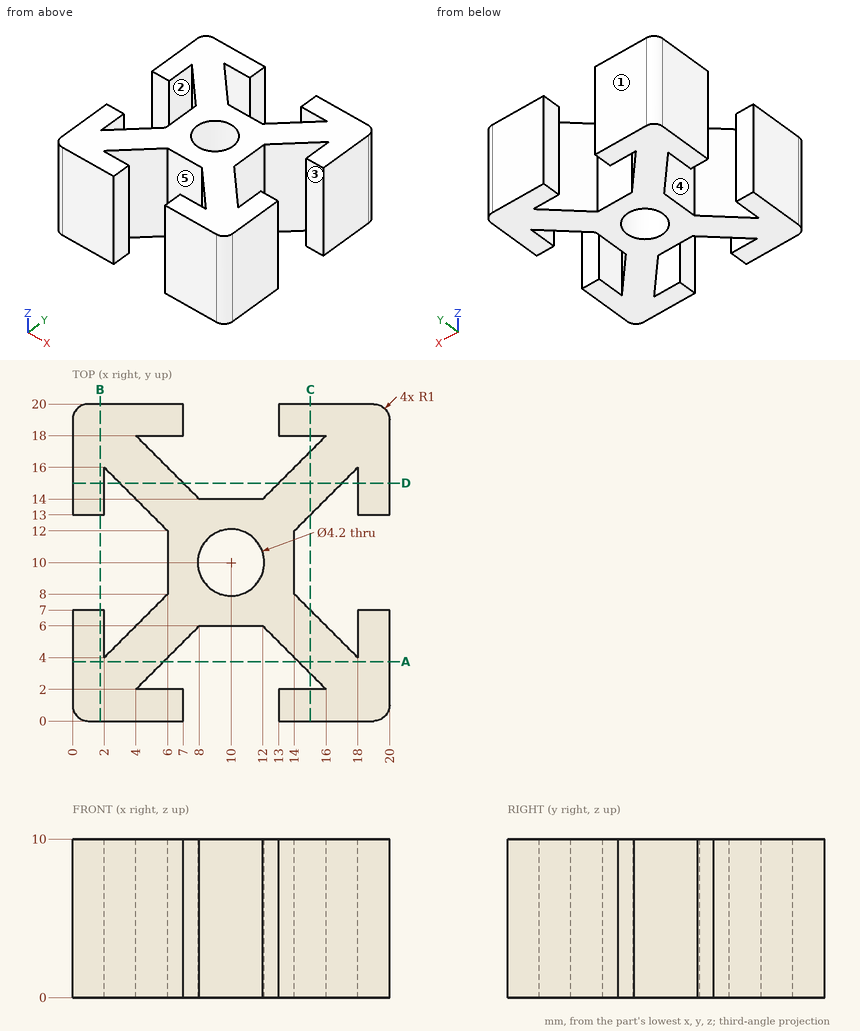
The figure shows three views and two pictorial views of one solid part (mm, origin at its lowest corner). Answer the questions. A direction names the side the tool comes from. Give positions to 0.01 mm unless a question says otherwise; leave off trailing zeros. Write each loop counter-clockwise with the first axis right and the second up, starting at its lowest first coordinate (ties: lowest second). Pieces come first, ordered by that corner, then holes. Notation, with made-up numbers: (12.25, -16.75) - (50.25, -16.75) arc R25 cw to (50.25, 19.25) - close; hole circle Ø7 at (44.25, 44.5). An arc over 180 degrees is marked (long way). Return JSON: item names as keys, results as strings.
Q1. A cutting plane is placed at A-A, the plane y = 3.75. Determine the outline of the cut face in (x, z).
Reply:
{"outline": "(0, 0) - (5.75, 0) - (5.75, 10) - (0, 10) - close; (14.25, 0) - (20, 0) - (20, 10) - (14.25, 10) - close"}
Q2. A cutting plane is placed at B-B, the plane x = 1.75. Determine the outline of the cut face in (y, z).
Reply:
{"outline": "(0, 0) - (7, 0) - (7, 10) - (0, 10) - close; (13, 0) - (20, 0) - (20, 10) - (13, 10) - close"}
Q3. A cutting plane is placed at C-C, the plane x = 15. Determine the outline of the cut face in (y, z).
Reply:
{"outline": "(0, 0) - (2, 0) - (2, 10) - (0, 10) - close; (3, 0) - (7, 0) - (7, 10) - (3, 10) - close; (13, 0) - (17, 0) - (17, 10) - (13, 10) - close; (18, 0) - (20, 0) - (20, 10) - (18, 10) - close"}
Q4. Consider line 1 along X through (y, z) = (5.25, 9.75); line 2 along Y through (x, z) = (15.25, 4.5). Determine where each line is inside the solid, lowest interval first. Write a range as [from, to].
Reply:
{"line 1": "[0, 2], [3.25, 7.25], [12.75, 16.75], [18, 20]", "line 2": "[0, 2], [2.75, 6.75], [13.25, 17.25], [18, 20]"}
Q5. For the marked faces 1, 2, 3, 4 and 5, determine the directions among +Z, -Z, +X, -X, +Y, -Y from which every point of the face is accessible in a straight line to the end or side of a thin tool.
Reply:
{"face 1": "+Z, -Z, +X, -X, +Y", "face 2": "+Z, -Z", "face 3": "+Z, -Z, +X", "face 4": "+Z, -Z, -X", "face 5": "+Z, -Z, -Y"}
Q6. Given P1, Ø0.6, axis at y = 0.5, z = 6, coming from the +X side; P2, Ø12, axis at x = 6, y = 7, coming from the -Z side; P3, Ø4.5, axis at x = 10.5, z = 6, coming from the -Y side; P4, Ø4.5, axis at x = 10, z = 4, coming from the +Y side, each flat-ended and moving along its own axis, determine where each tip first touches the part or whether it passes through.
Reply:
{"P1": "x = 19.98", "P2": "z = 0", "P3": "y = 5.25", "P4": "y = 14.25"}
